Input: part model. Units: mm. Frame: model coordinates. Coordinates: 2 decimals unless noted, no trailing zeros. Loops run counter-clockwise (first coordinate to the right, second up) from the corner with the lowest first, then second, coordinate; pieces in that order, holes last.
```python
from build123d import *

# Parameters (mm, degrees)
BOSS_EXTRUDE1_DEPTH = 5
SKETCH2_R           = 7.95
CUT_EXTRUDE3_DEPTH  = 5
SKETCH4_R           = 2.5
SKETCH4_R_2         = 5.925
CUT_EXTRUDE4_DEPTH  = 5


with BuildPart() as part:
    # Sketch1 → Boss-Extrude1 (new body)
    with BuildSketch(Plane(origin=(0, 0, 0), x_dir=(1, 0, 0), z_dir=(0, 1, 0))):
        with BuildLine():
            Line((-34.721115538, 28.398406375), (31.278884462, 28.398406375))
            ThreePointArc((31.278884462, 28.398406375), (33.400204806, 27.519726718), (34.278884462, 25.398406375))
            Line((34.278884462, 25.398406375), (34.278884462, -50.601593625))
            ThreePointArc((34.278884462, -50.601593625), (33.400204806, -52.722913969), (31.278884462, -53.601593625))
            Line((31.278884462, -53.601593625), (-34.721115538, -53.601593625))
            ThreePointArc((-34.721115538, -53.601593625), (-36.842435881, -52.722913969), (-37.721115538, -50.601593625))
            Line((-37.721115538, -50.601593625), (-37.721115538, 25.398406375))
            ThreePointArc((-37.721115538, 25.398406375), (-36.842435881, 27.519726718), (-34.721115538, 28.398406375))
        make_face()
    extrude(amount=BOSS_EXTRUDE1_DEPTH)

    # Sketch2 → Cut-Extrude3 (cut)
    with BuildSketch(Plane(origin=(0, 5, 0), x_dir=(1, 0, 0), z_dir=(0, 1, 0))):
        with Locations(Location((-14.996537264, 0, 0), (0, 0, 270))):
            Circle(SKETCH2_R)
        with Locations(Location((9.453462736, 0, 0), (0, 0, 270))):
            Circle(SKETCH2_R)
    extrude(amount=-CUT_EXTRUDE3_DEPTH, mode=Mode.SUBTRACT)

    # Sketch4 → Cut-Extrude4 (cut)
    with BuildSketch(Plane(origin=(0, 5, 0), x_dir=(1, 0, 0), z_dir=(0, 1, 0))):
        with Locations(Location((-2.024594695, -12.601593625, 0), (0, 0, 270))):
            Circle(SKETCH4_R)
        with Locations(Location((-2.139356247, -28.105866385, 0), (0, 0, 270))):
            Circle(SKETCH4_R_2)
    extrude(amount=-CUT_EXTRUDE4_DEPTH, mode=Mode.SUBTRACT)


solid = part.part
```
Item 1: Line query: L1, parallel to X at y = 2.65, z = 0; L2, parallel to Z at x = -4, y = 3.9; L3, parallel to X at y = 3.15, z = 6.5. Output: solid intervals per line, ascending.
Result:
L1: x = -37.72 to -22.95, -7.05 to 1.5, 17.4 to 34.28
L2: z = -28.4 to 11.07, 14.13 to 22.48, 33.73 to 53.6
L3: x = -37.72 to -19.57, -10.42 to 4.88, 14.03 to 34.28
Item 2: Contact query for flat-ended pins moving along their axis: P1, Ø14.5, axis at x = 9.45, z = 0, coming from the +Y side; P2, Ø8, axis at x = 20, z = 15, coming from the -Y side. Output: stop coordinate, or through.
Result:
P1: passes through
P2: stops at y = 0
Item 3: Section query C-C (x = 10.5). Output: boundary loops of the cut face in (y, z), then the cut area to 3 significant figures.
Result:
outline: (0, -28.4) - (5, -28.4) - (5, -7.88) - (0, -7.88) - close; (0, 7.88) - (5, 7.88) - (5, 53.6) - (0, 53.6) - close
area: 331 mm2
Item 4: Section query A-A (z = 0). Output: boundary loops of the cut face in (x, y).
Result:
outline: (-37.72, 0) - (-22.95, 0) - (-22.95, 5) - (-37.72, 5) - close; (-7.05, 0) - (1.5, 0) - (1.5, 5) - (-7.05, 5) - close; (17.4, 0) - (34.28, 0) - (34.28, 5) - (17.4, 5) - close
Item 5: Section query D-D (y = 2.45). Output: boundary loops of the cut face in (x, z) (3 decimals).
Result:
outline: (-37.721, -25.398) arc R3 ccw to (-34.721, -28.398) - (31.279, -28.398) arc R3 ccw to (34.279, -25.398) - (34.279, 50.602) arc R3 ccw to (31.279, 53.602) - (-34.721, 53.602) arc R3 ccw to (-37.721, 50.602) - close; hole circle Ø15.9 at (-14.997, 0); hole circle Ø11.85 at (-2.139, 28.106); hole circle Ø5 at (-2.025, 12.602); hole circle Ø15.9 at (9.453, 0)
Item 6: Section query B-B (z = 27.5). Output: boundary loops of the cut face in (x, y), then the cut area to 3 significant figures.
Result:
outline: (-37.72, 0) - (-8.03, 0) - (-8.03, 5) - (-37.72, 5) - close; (3.75, 0) - (34.28, 0) - (34.28, 5) - (3.75, 5) - close
area: 301 mm2
